```python
from build123d import *

# Parameters (mm, degrees)
SKETCH3_W           = 5.48566609
SKETCH3_H           = 3.701966347
SKETCH3_W_2         = 2.548907401
SKETCH3_H_2         = 5.128177147
BOSS_EXTRUDE2_DEPTH = 10
FILLET1_R           = 2


with BuildPart() as part:
    # Sketch3 → Boss-Extrude2 (new body)
    with BuildSketch(Plane.XY):
        with Locations((2.742833045, 1.850983174)):
            Rectangle(SKETCH3_W, SKETCH3_H)
        with Locations((2.68186795, -2.564088574)):
            Rectangle(SKETCH3_W_2, SKETCH3_H_2)
    extrude(amount=BOSS_EXTRUDE2_DEPTH)

    # Fillet1
    # the kernel refuses this fillet: 2 mm, written as the material it adds along each edge
    with BuildSketch(Plane(origin=(3.95632165, 0, 0), x_dir=(1, 0, 0), z_dir=(0, 0, 1))) as fillet1_piece_1:
        with BuildLine():
            CenterArc((2, -1.943832129), FILLET1_R, 103.610945059, 76.389054941)
            Line((0, -1.943832129), (-0.04, -1.943832129))
            Line((-0.04, -1.943832129), (-0.04, 0))
            Line((-0.04, 0), (0, 0.04))
            ThreePointArc((0, 0.04), (0.76467222, 0.04), (1.519931329, 0.038876643))
            Line((1.519931329, 0.038876643), (1.52934444, 0))
        make_face()
    extrude(amount=10)
    with BuildSketch(Plane(origin=(1.407414249, 0, 0), x_dir=(-1, 0, 0), z_dir=(0, 0, 1))) as fillet1_piece_2:
        with BuildLine():
            CenterArc((2, 1.910194265), FILLET1_R, 180, 72.764919968)
            Line((0, 1.910194265), (-0.04, 1.910194265))
            Line((-0.04, 1.910194265), (-0.04, 0))
            Line((-0.04, 0), (0, -0.04))
            ThreePointArc((0, -0.04), (0.703707125, -0.04), (1.395562534, -0.038203885))
            Line((1.395562534, -0.038203885), (1.407414249, 0))
        make_face()
    extrude(amount=10)


solid = part.part
```
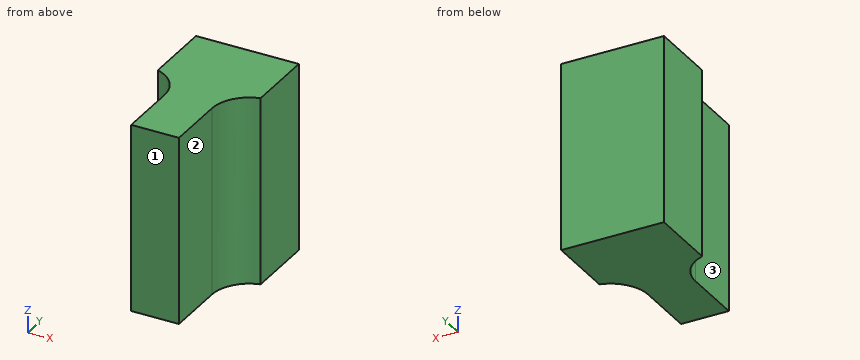
Source: CAD feature listing. Evaluate the final solid. Frame: model axes, mm. Face numbers are marked on the shaded views. A direction names the side the tool comes from. Coordinates: 2 decimals unless noted, no trailing zeros. Write each loop counter-clockwise with the first axis right and the second up, starting at its lowest first coordinate (ties: lowest second). Pieces come first, ordered by that corner, then holes. Notation, with made-up numbers: (-8, 83) - (22, 83) arc R25 ccw to (22, 117) - close; hole circle Ø11 at (-28.5, 46). An arc over 180 degrees is marked (long way). Answer as a JSON object with one key per item and string values.
Q1. First-contact query: pin 1 Ø2 at (y, z) = (-2, 8.5) entering from -X; pin 2 Ø3.5 at (y, z) = (-3, 6.5) entering from +X; pin 3 Ø4 at (y, z) = (-3.5, 4.5) entering from +X. Flat tips, straight axial feed; report the tip coordinate or a pass-through.
Ans:
{"pin 1": "stops at x = 1.19", "pin 2": "stops at x = 4.08", "pin 3": "stops at x = 4.01"}
Q2. Section query C-C, the plane x = 0.5. Output: boundary loops of the cut face in (y, z) (3 decimals), plus the area to 3 significant figures.
Ans:
{"outline": "(-0.235, 0) - (3.702, 0) - (3.702, 10) - (-0.235, 10) - close", "area": "39.4 mm2"}
Q3. Section query B-B, the plane y = -4. Output: boundary loops of the cut face in (x, z), plus the area to 3 significant figures.
Ans:
{"outline": "(1.41, 0) - (3.96, 0) - (3.96, 10) - (1.41, 10) - close", "area": "25.5 mm2"}
Q4. Set-up query: the marked faces 1, 2 and 3. Return all of +Z, -Z, +X, -X, +Y, -Y with unobstructed straight access to the full face (end or side cutting, diameter ignored); none if empty.
Ans:
{"face 1": "+Z, -Z, +X, -X, -Y", "face 2": "+Z, -Z, +X, -Y", "face 3": "+Z, -Z, -X, -Y"}
Q5. Material intervals for line 1 (X direction, y = -2.25, z = 1.75); line 2 (Y direction, x = 0.35, z = 3.5); line 3 (X direction, y = -1, z = 4.5), sorted ascending. Write a range as [from, to].
Ans:
{"line 1": "x = [1.41, 3.96]", "line 2": "y = [-0.15, 3.7]", "line 3": "x = [1.19, 4.19]"}
Q6. Section query A-A, the plane z = 4. Output: boundary loops of the cut face in (x, y), plus the area to 3 significant figures.
Ans:
{"outline": "(0, 0) arc R2 cw to (1.41, -1.91) - (1.41, -5.13) - (3.96, -5.13) - (3.96, -1.94) arc R2 cw to (5.49, 0) - (5.49, 3.7) - (0, 3.7) - close", "area": "34.9 mm2"}
